```python
from build123d import *

# Parameters (mm, degrees)
SKETCH3_R                = 6
BOSS_EXTRUDE2_DEPTH      = 100
BOSS_EXTRUDE2_DEPTH_BACK = 100
CUT_EXTRUDE5_DEPTH       = 101
CUT_EXTRUDE5_DEPTH_BACK  = 101
CHAMFER1_SIZE            = 0.6


with BuildPart() as part:
    # Sketch3 → Boss-Extrude2 (new body, two sides)
    with BuildSketch(Plane.XY) as boss_extrude2_sk:
        Circle(SKETCH3_R)
    extrude(amount=BOSS_EXTRUDE2_DEPTH)
    extrude(boss_extrude2_sk.sketch, amount=-BOSS_EXTRUDE2_DEPTH_BACK)

    # Sketch10 → Cut-Extrude5 (cut, two sides)
    with BuildSketch(Plane.XY) as cut_extrude5_sk:
        with BuildLine():
            Line((-3, 5.196152423), (3, 5.196152423))
            ThreePointArc((3, 5.196152423), (0, 6), (-3, 5.196152423))
        make_face()
    extrude(amount=CUT_EXTRUDE5_DEPTH, mode=Mode.SUBTRACT)
    extrude(cut_extrude5_sk.sketch, amount=-CUT_EXTRUDE5_DEPTH_BACK, mode=Mode.SUBTRACT)

    # Chamfer1
    chamfer1_edges = [part.edges().sort_by_distance(p)[0] for p in [
        (0, -6, -100),
        (0, -6, 100),
    ]]
    chamfer(chamfer1_edges, length=CHAMFER1_SIZE)


solid = part.part
```
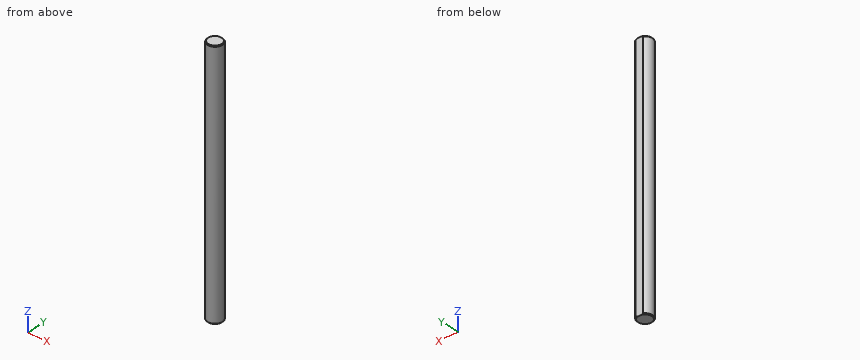
Design review of the part built by this model. Coordinates are the model's own, in mm. Round coordinates to 2 decimals unless told otherwise and drop trailing zeros. Order: outer loops, then holes, each group sorted by start corner. A loop starts at its lowest first (then second) coordinate and runs counter-clockwise, first axis right, second up. Notation, with made-up numbers: M 2,-26.75 L 39,-26.75 A20 ccw 39,-16.75 Z; hole C -11.5,28.25 d5. An arc over 180 degrees is marked long. Put each result on its own line as item: value.
Q1. Insertion check: pin 1 Ø4 at (x, z) = (-3.5, -46.5) entering from +Y; pin 2 Ø1 at (y, z) = (-2.5, 45.5) entering from -X; pin 3 Ø5 at (x, z) = (-3, 9) entering from -Y; pin 4 Ø3 at (x, z) = (-3, -67.5) entering from -Y. Each pin has a flat end and moves straight along its axis. Give the tip position at first contact, or say it passes through.
Reported:
pin 1: y = 5.2
pin 2: x = -5.66
pin 3: y = -5.98
pin 4: y = -5.81
Q2. Consider section A-A (z = -17.5). State the section outline as (x, y) points.
Reported:
outline: M -3,5.2 A6 ccw long 3,5.2 Z
Q3. To check wall thickness, follow line 1 (Y direction, x = 0.25, z = 69); line 2 (X direction, y = 0.5, z = 60); line 3 (Y direction, x = 1, z = -8.5). State the ranges of each line that lie inside material, in increasing order.
Reported:
line 1: -5.99 to 5.2
line 2: -5.98 to 5.98
line 3: -5.92 to 5.2
